from build123d import *

# Parameters (mm, degrees)
SKETCH_2_R      = 1.3
SKETCH_2_R_2    = 4
SKETCH_2_R_3    = 1.925
EXTRUDE_1_DEPTH = 1.5


with BuildPart() as part:
    # 草圖2 → 填料-伸長1 (new body)
    with BuildSketch(Plane(origin=(0, 0, 0), x_dir=(0, 0, -1), z_dir=(1, 0, 0))):
        with BuildLine():
            Line((18.012072511, -21.441606673), (11.718522882, 46.276737912))
            ThreePointArc((11.718522882, 46.276737912), (1.55399875, 55.843411078), (-8.930005845, 46.627965677))
            Line((-8.930005845, 46.627965677), (-17.523002046, -20.837161438))
            ThreePointArc((-17.523002046, -20.837161438), (-18.27264724, -25.183298229), (-19.402359762, -29.446468708))
            ThreePointArc((-19.402359762, -29.446468708), (-19.752456192, -30.70663404), (-20.020797275, -31.986703271))
            ThreePointArc((-20.020797275, -31.986703271), (-0.345749536, -55.841970902), (20.12922907, -32.669648007))
            ThreePointArc((20.12922907, -32.669648007), (19.904578122, -31.38119307), (19.597542195, -30.109850035))
            ThreePointArc((19.597542195, -30.109850035), (18.61347279, -25.810724505), (18.012072511, -21.441606673))
        make_face()
        with Locations((-6.388480657, -35.515504866)):
            Circle(SKETCH_2_R, mode=Mode.SUBTRACT)
        with Locations((0.111519343, -42.015504866)):
            Circle(SKETCH_2_R, mode=Mode.SUBTRACT)
        with Locations((0, -35.515504866)):
            Circle(SKETCH_2_R_2, mode=Mode.SUBTRACT)
        with Locations((0.111519343, -29.015504866)):
            Circle(SKETCH_2_R, mode=Mode.SUBTRACT)
        with Locations((6.611519343, -35.515504866)):
            Circle(SKETCH_2_R, mode=Mode.SUBTRACT)
        with Locations((1.377596172, 45.472779649)):
            Circle(SKETCH_2_R_3, mode=Mode.SUBTRACT)
    extrude(amount=EXTRUDE_1_DEPTH)


solid = part.part
Here's how the part is built. I have some questions about the finished solid (model axes, mm). Give positions to 0.01 mm unless a question says otherwise; leave off trailing zeros. Loops run counter-clockwise (first coordinate to the right, second up) from the corner with the lowest first, then second, coordinate; pieces in that order, holes last. Notation, with made-up numbers: (62, -15.75) -> (77, -15.75) arc R33 ccw to (77, 18.25) -> close; hole circle Ø1 at (47.5, 62.5). An arc over 180 degrees is marked (long way). Answer as a JSON object with one key per item and string values. Group by question number.
Item 1: Imagine slicing it at C-C on z = 14. Write out the boundary of the cut face in (x, y).
Item 2: Thinking about a two-plate mould opening in Y: for faces 1 (the flat face through (0.74, 11.94, -14.91)), 2 (the cylindrical face through (0.74, -36.785, 6.67)), 3 (the flat face through (1.5, 1, 0)), which applies, pulls with the +Y half, pulls with the -Y half, needs draft (parallel to the pull), parting line crosses it, or undercut?
Item 3: Imagine slicing it at B-B on y = 31. Write out the boundary of the cut face in (x, z), then the cut area to 3 significant figures.
Item 4: I need wall thicknesses on L1, parallel to Z at x = 0.75, y = -35.5; L2, parallel to Y at x = 0.7, z = 0; L3, parallel to Y at x = 0.7, z = -1.5. Which ranges of each line are inside material? Lowest first, please.
Item 5: Imagine slicing it at A-A on x = 1.1. Give the number of separate pieces and of enclosed holes in the cut face, then the cut area to 3 significant figures.
Answer list:
{
 "1": {"outline": "(0, -50.26) -> (1.5, -50.26) -> (1.5, 6.82) -> (0, 6.82) -> close"},
 "2": {"face 1": "pulls with the +Y half", "face 2": "undercut", "face 3": "needs draft"},
 "3": {"outline": "(0, -13.14) -> (1.5, -13.14) -> (1.5, 10.92) -> (0, 10.92) -> close", "area": "36.1 mm2"},
 "4": {"L1": "z = -20.33 to -7.91, -5.31 to -4, 4 to 5.09, 7.69 to 20.33", "L2": "y = -55.84 to -43.31, -40.72 to -39.52, -31.52 to -30.31, -27.72 to 44.13, 46.82 to 55.75", "L3": "y = -55.79 to -39.22, -31.81 to 43.55, 47.39 to 55.84"},
 "5": {"separate pieces": "1", "enclosed holes": "6", "area": "3,160 mm2"}
}
